```python
from build123d import *

# Parameters (mm, degrees)
SKETCH1_W           = 50
SKETCH1_H           = 50
SKETCH1_W_2         = 45.6
SKETCH1_H_2         = 45.6
BOSS_EXTRUDE1_DEPTH = 1923
SKETCH2_W           = 40
SKETCH2_H           = 50
CUT_EXTRUDE2_DEPTH  = 50


with BuildPart() as part:
    # Sketch1 → Boss-Extrude1 (new body)
    with BuildSketch(Plane(origin=(0, 0, 0), x_dir=(1, 0, 0), z_dir=(0, 1, 0))):
        with Locations((25, 25)):
            Rectangle(SKETCH1_W, SKETCH1_H)
        with Locations((25, 25)):
            Rectangle(SKETCH1_W_2, SKETCH1_H_2, mode=Mode.SUBTRACT)
    extrude(amount=BOSS_EXTRUDE1_DEPTH)

    # Sketch2 → Cut-Extrude2 (cut)
    with BuildSketch(Plane.XY):
        with Locations((20, 25)):
            Rectangle(SKETCH2_W, SKETCH2_H)
        with Locations((20, 1898)):
            Rectangle(SKETCH2_W, SKETCH2_H)
    extrude(amount=-CUT_EXTRUDE2_DEPTH, mode=Mode.SUBTRACT)


solid = part.part
```
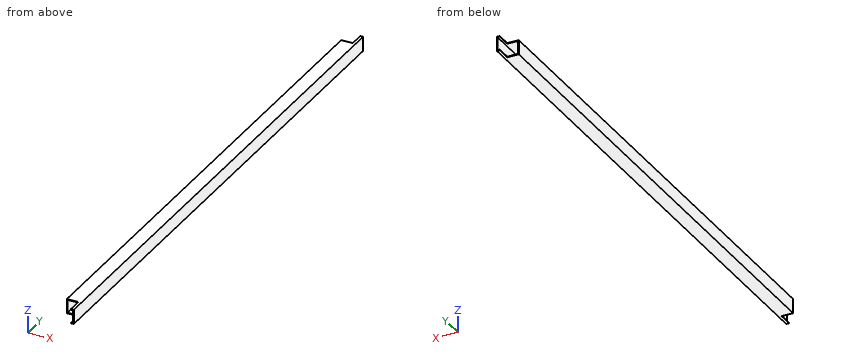
Work out the finished part from the listing and answer in its coordinate system (mm). Give positions to 0.01 mm unless a question says otherwise; leave off trailing zeros. Order: outer loops, then holes, each group sorted by start corner. A loop starts at its lowest first (then second) coordinate and runs counter-clockwise, first axis right, second up. Notation, with made-up numbers: (-20.5, -16.5) -> (13.5, -16.5) arc R26 ccw to (13.5, 4.5) -> close; hole circle Ø9 at (10.25, 57). An arc over 180 degrees is marked (long way). Answer as CSV lines item,"result". Start each with the question number.
(1) This flat-tipped pin is pushed along its axis until it touches: pin 1 Ø1.1 at (y, z) = (31.5, -1.5) entering from -X. Where does it stop, or does it pass through?
(2) Section C-C, the plane x = 20.5 is taken. Write down the section's boundary in (y, z), plus the area to 3 significant figures.
(3) Consider line 1 along X through (y, z) = (644, -6); line 2 along Z through (x, y) = (3, 1676.5); line 3 along Y through (x, z) = (25, -2). Determine where each line is inside the solid, lowest interval first.
(4) Section B-B, the plane y = 1666 is taken. Write down the section's boundary in (x, z).
(5) Section A-A, the plane z = -19 is taken. Write down the section's boundary in (x, y), plus the area to 3 significant figures.
Entries:
1,pin 1,"x = 40"
2,outline,"(50, -50) -> (1873, -50) -> (1873, -47.8) -> (50, -47.8) -> close; (50, -2.2) -> (1873, -2.2) -> (1873, 0) -> (50, 0) -> close"
2,area,"8,020 mm²"
3,line 1,"0 to 2.2, 47.8 to 50"
3,line 2,"-50 to -47.8, -2.2 to 0"
3,line 3,"50 to 1873"
4,outline,"(0, -50) -> (50, -50) -> (50, 0) -> (0, 0) -> close; hole (2.2, -47.8) -> (47.8, -47.8) -> (47.8, -2.2) -> (2.2, -2.2) -> close"
5,outline,"(0, 50) -> (2.2, 50) -> (2.2, 1873) -> (0, 1873) -> close; (47.8, 0) -> (50, 0) -> (50, 1923) -> (47.8, 1923) -> close"
5,area,"8,240 mm²"
